CAD build for the part. Positions are in the model's coordinates, mm. A direction names the side the tool comes from. Give positions to 0.01 mm unless a question says otherwise; leave off trailing zeros. Order: outer loops, then holes, each group sorted by start corner. A loop starts at its lowest first (then second) coordinate and runs counter-clockwise, first axis right, second up. Notation, with made-up numbers: (33, 48.25) -> (82, 48.25) arc R15 ccw to (82, 70.25) -> close; hole circle Ø6 at (17.5, 66.5). An arc over 180 degrees is marked (long way). Answer as CSV lines item,"result".
```python
from build123d import *

# Parameters (mm, degrees)
RESSALTO_EXTRUS_O1_DEPTH = 5
ESBO_O2_R                = 2.5
CORTE_EXTRUS_O1_DEPTH    = 5
RESSALTO_EXTRUS_O3_DEPTH = 35
CORTE_EXTRUS_O2_DEPTH    = 10
ESBO_O7_W                = 55
ESBO_O7_H                = 5
RESSALTO_EXTRUS_O4_DEPTH = 20
ESBO_O8_W                = 55
ESBO_O8_H                = 5
ESBO_O8_H_2              = 5.000335185
RESSALTO_EXTRUS_O6_DEPTH = 105
ESBO_O9_W                = 7.5
ESBO_O9_H                = 20
CORTE_EXTRUS_O4_DEPTH    = 5
ESBO_O10_W               = 7.5
ESBO_O10_H               = 20
CORTE_EXTRUS_O5_DEPTH    = 5
ESBO_O11_W               = 105
ESBO_O11_H               = 5.000335185
CORTE_EXTRUS_O6_DEPTH    = 10
ESBO_O12_W               = 105
ESBO_O12_H               = 5.000335185
CORTE_EXTRUS_O7_DEPTH    = 10
ESBO_O13_W               = 105
ESBO_O13_H               = 5.000335185
CORTE_EXTRUS_O8_DEPTH    = 10
ESBO_O14_W               = 105
ESBO_O14_H               = 5.000335185
CORTE_EXTRUS_O9_DEPTH    = 10


with BuildPart() as part:
    # Esboço1 → Ressalto-extrusão1 (new body)
    with BuildSketch(Plane(origin=(0, 0, 0), x_dir=(1, 0, 0), z_dir=(0, 1, 0))):
        with BuildLine():
            Line((140, -100), (-90, -100))
            ThreePointArc((-90, -100), (-97.071067812, -97.071067812), (-100, -90))
            Line((-100, -90), (-100, 90))
            ThreePointArc((-100, 90), (-97.071067812, 97.071067812), (-90, 100))
            Line((-90, 100), (140, 100))
            ThreePointArc((140, 100), (147.071067812, 97.071067812), (150, 90))
            Line((150, 90), (150, -90))
            ThreePointArc((150, -90), (147.071067812, -97.071067812), (140, -100))
        make_face()
    extrude(amount=RESSALTO_EXTRUS_O1_DEPTH)

    # Esboço2 → Corte-extrusão1 (cut)
    with BuildSketch(Plane(origin=(0, 5, 0), x_dir=(1, 0, 0), z_dir=(0, 1, 0))):
        with Locations(Location((-85, 85, 0), (0, 0, 270))):
            Circle(ESBO_O2_R)
        with Locations(Location((-10, -85, 0), (0, 0, 270))):
            Circle(ESBO_O2_R)
        with Locations(Location((60, -85, 0), (0, 0, 270))):
            Circle(ESBO_O2_R)
        with Locations(Location((135, 85, 0), (0, 0, 270))):
            Circle(ESBO_O2_R)
    extrude(amount=-CORTE_EXTRUS_O1_DEPTH, mode=Mode.SUBTRACT)

    # Esboço5 → Ressalto-extrusão3 (add)
    with BuildSketch(Plane(origin=(0, 5, 0), x_dir=(1, 0, 0), z_dir=(0, 1, 0))):
        Polygon((125, -55), (105, -55), (105, 50), (125, 50), (130, 50), (130, 55), (75, 55), (75, 50), (80, 50), (100, 50), (100, -55), (80, -55), (75, -55), (75, -60), (130, -60), (130, -55), align=None)
        Polygon((-50, -55), (-50, 50), (-30, 50), (-25, 50), (-25, 55), (-80, 55), (-80, 50), (-75, 50), (-55, 50), (-55, -55), (-75, -55), (-80, -55), (-80, -60), (-25, -60), (-25, -55), (-30, -55), align=None)
    extrude(amount=RESSALTO_EXTRUS_O3_DEPTH)

    # Esboço6 → Corte-extrusão2 (cut)
    with BuildSketch(Plane(origin=(0, 5, 0), x_dir=(1, 0, 0), z_dir=(0, 1, 0))):
        with BuildLine():
            Line((23.718326371, 50), (26.281673629, 50))
            ThreePointArc((26.281673629, 50), (46.58859695, 41.58859695), (55, 21.281673629))
            Line((55, 21.281673629), (55, -21.281673629))
            ThreePointArc((55, -21.281673629), (46.58859695, -41.58859695), (26.281673629, -50))
            Line((26.281673629, -50), (23.718326371, -50))
            ThreePointArc((23.718326371, -50), (3.41140305, -41.58859695), (-5, -21.281673629))
            Line((-5, -21.281673629), (-5, 21.281673629))
            ThreePointArc((-5, 21.281673629), (3.41140305, 41.58859695), (23.718326371, 50))
        make_face()
    extrude(amount=-CORTE_EXTRUS_O2_DEPTH, mode=Mode.SUBTRACT)

    # Esboço7 → Ressalto-extrusão4 (add)
    with BuildSketch(Plane(origin=(0, 40, 0), x_dir=(1, 0, 0), z_dir=(0, 1, 0))):
        with Locations((102.5, -57.5)):
            Rectangle(ESBO_O7_W, ESBO_O7_H)
        with Locations((102.5, 52.5)):
            Rectangle(ESBO_O7_W, ESBO_O7_H)
        with Locations((-52.5, 52.5)):
            Rectangle(ESBO_O7_W, ESBO_O7_H)
        with Locations((-52.5, -57.5)):
            Rectangle(ESBO_O7_W, ESBO_O7_H)
    extrude(amount=RESSALTO_EXTRUS_O4_DEPTH)

    # Esboço8 → Ressalto-extrusão6 (add)
    with BuildSketch(Plane.XY.offset(-50)):
        with Locations((102.5, 57.5)):
            Rectangle(ESBO_O8_W, ESBO_O8_H)
        with Locations((-52.5, 57.5)):
            Rectangle(ESBO_O8_W, ESBO_O8_H)
        with Locations((102.5, 42.500167593)):
            Rectangle(ESBO_O8_W, ESBO_O8_H_2)
        with Locations((-52.5, 42.500167593)):
            Rectangle(ESBO_O8_W, ESBO_O8_H_2)
    extrude(amount=RESSALTO_EXTRUS_O6_DEPTH)

    # Esboço9 → Corte-extrusão4 (cut)
    with BuildSketch(Plane(origin=(0, 0, -55), x_dir=(-1, 0, 0), z_dir=(0, 0, -1))):
        with Locations((-96.25, 15)):
            Rectangle(ESBO_O9_W, ESBO_O9_H)
        with Locations((58.75, 15)):
            Rectangle(ESBO_O9_W, ESBO_O9_H)
    extrude(amount=-CORTE_EXTRUS_O4_DEPTH, mode=Mode.SUBTRACT)

    # Esboço10 → Corte-extrusão5 (cut)
    with BuildSketch(Plane.XY.offset(60)):
        with Locations((-46.25, 15)):
            Rectangle(ESBO_O10_W, ESBO_O10_H)
        with Locations((108.75, 15)):
            Rectangle(ESBO_O10_W, ESBO_O10_H)
    extrude(amount=-CORTE_EXTRUS_O5_DEPTH, mode=Mode.SUBTRACT)

    # Esboço11 → Corte-extrusão6 (cut)
    with BuildSketch(Plane(origin=(130, 0, 0), x_dir=(0, 0, -1), z_dir=(1, 0, 0))):
        with Locations((-2.5, 42.500167593)):
            Rectangle(ESBO_O11_W, ESBO_O11_H)
    extrude(amount=-CORTE_EXTRUS_O6_DEPTH, mode=Mode.SUBTRACT)

    # Esboço12 → Corte-extrusão7 (cut)
    with BuildSketch(Plane.ZY.offset(-75)):
        with Locations((2.5, 42.500167593)):
            Rectangle(ESBO_O12_W, ESBO_O12_H)
    extrude(amount=-CORTE_EXTRUS_O7_DEPTH, mode=Mode.SUBTRACT)

    # Esboço13 → Corte-extrusão8 (cut)
    with BuildSketch(Plane(origin=(-25, 0, 0), x_dir=(0, 0, -1), z_dir=(1, 0, 0))):
        with Locations((-2.5, 42.500167593)):
            Rectangle(ESBO_O13_W, ESBO_O13_H)
    extrude(amount=-CORTE_EXTRUS_O8_DEPTH, mode=Mode.SUBTRACT)

    # Esboço14 → Corte-extrusão9 (cut)
    with BuildSketch(Plane.ZY.offset(80)):
        with Locations((2.5, 42.500167593)):
            Rectangle(ESBO_O14_W, ESBO_O14_H)
    extrude(amount=-CORTE_EXTRUS_O9_DEPTH, mode=Mode.SUBTRACT)


solid = part.part
```
1) Pin check, flat tips, straight feed: P1, Ø1.5, axis at x = -39.5, y = 35.5, coming from the +Z side; P2, Ø5, axis at x = -9, z = 52, coming from the +Y side; P3, Ø4, axis at y = 19, z = 58, coming from the -X side. Stop position of each tip, or through.
Data:
P1,"stops at z = 60"
P2,"stops at y = 5"
P3,"stops at x = -80"
2) Band-saw the part on C-C, the plane x = 13. Write the cut outline in (y, z), then the cut area to 3 significant figures.
Data:
outline,"(0, -100) -> (5, -100) -> (5, -47.92) -> (0, -47.92) -> close; (0, 47.92) -> (5, 47.92) -> (5, 100) -> (0, 100) -> close"
area,"521 mm2"
3) Which spindle directions (+Z, -Z, +X, -X, +Y, -Y) get a long thin tool onto all of the face, cutting with end or side? Do faces 1 (the flat face through (-53, 55, 2)), 2 (the flat face through (-46, 25, 58)), 3 (the flat face through (-62.5, 15, -53)). Say none if no direction does.
Data:
face 1,"+X, -X"
face 2,"+Z"
face 3,"-Z"
4) Pull direction X, two halves, no side cores. Call faces 4 (the flat face through (75, 57, 2)), 5 (the cylindrical face through (-97.15, 2.46, -96.99)), 6 (the flat face through (102, 55, 2)), 7 (the flat face through (112.5, 15, 58)): pulls with the +X half, pulls with the -X half, needs draft (parallel to the pull), parting line crosses it, or undercut.
Data:
face 4,"undercut"
face 5,"pulls with the -X half"
face 6,"needs draft"
face 7,"undercut"
5) Band-saw the part on D-D, the plane z = 63. Write the cut outline in (x, y), then the cut area to 3 significant figures.
Data:
outline,"(-100, 0) -> (150, 0) -> (150, 5) -> (-100, 5) -> close"
area,"1,250 mm2"
6) Band-saw the part on A-A, the plane y = 12. Give the number of separate pieces and of enclosed holes in the cut face, then the cut area to 3 significant figures.
Data:
separate pieces,"6"
enclosed holes,"0"
area,"2,000 mm2"
7) Wall check: line 1 along X through (y, z) = (2, 85); line 2 along Y through (x, z) = (96.5, 32.5); line 3 along Y through (x, z) = (82, -21). Give the ranges that are in metal, low to high. Write a range as [from, to].
Data:
line 1,"x = [-100, -12.5], [-7.5, 57.5], [62.5, 150]"
line 2,"y = [0, 5], [40, 45], [55, 60]"
line 3,"y = [0, 5], [55, 60]"
